The model under review builds one solid part; all positions refer to its coordinate system, in mm. Round coordinates to 2 decimals unless told otherwise and drop trailing zeros. Loops run counter-clockwise (first coordinate to the right, second up) from the corner with the lowest first, then second, coordinate; pieces in that order, holes last. Notation, with made-up numbers: M 62.25,35 L 94.25,35 A3 cw 94.25,40 Z; hole C -24.5,57.5 d5. An arc over 180 degrees is marked long. Answer as a JSON object with one key per item and string values. Group by question number.
Item 1: Consider section C-C (y = 2). Give the boundary of the cut face in (x, z).
Item 2: Consider section D-D (z = 5.4). Give the boundary of the cut face in (x, y) (3 decimals).
Item 3: Insertion check: P1, Ø1, axis at y = 5, z = 1, coming from the -X side; P2, Ø2, axis at y = 4.5, z = 1, coming from the +X side. Each pin has a flat end and moves straight along its axis. Give the tip position at first contact, or say it passes through.
Item 4: To check wall thickness, follow line 1 (Y direction, x = 20, z = 3.05); line 2 (X direction, y = -1.5, z = 0.9); line 3 (X direction, y = -1.25, z = 3.3). State the ranges of each line that lie inside material, in increasing order.
Item 5: Consider section B-B (z = 3.1). Give the boundary of the cut face in (x, y) (3 decimals).
Item 6: The part is to be moulded in two halves that separate along Y. For faces 1 (the face through (10.055, -1.684, 2.859)), 2 (the face through (-8.521, 0.035, 4.922)), 3 (the face through (27.229, 4.779, 5.114)), 4 (the face through (-8.5, -6.07, 2.01)), say which applies: +Y half, -Y half, draft (parallel to the pull), parting line (faces both ways), or undercut.
Item 7: Consider section A-A (y = 0). Give the boundary of the cut face in (x, z) (3 decimals).
Solid Edge part; units mm, degrees
sketch "Sketch1" plane through (0, 0, 0) normal (0, 0, 1) x (1, 0, 0)
  line L0 (-5, -7.5) -> (25, -7.5)
  arc A0 (25, -7.5) -> (30, -2.5) centre (25, -2.5) ccw
  line L1 (30, -2.5) -> (30, 2.5)
  arc A1 (25, 7.5) -> (30, 2.5) centre (25, 2.5) cw
  line L2 (25, 7.5) -> (-5, 7.5)
  arc A2 (-10, 2.5) -> (-5, 7.5) centre (-5, 2.5) cw
  line L3 (-10, 2.5) -> (-10, -2.5)
  arc A3 (-10, -2.5) -> (-5, -7.5) centre (-5, -2.5) ccw
  arc A4 (1.1832, 1.15) -> (-1.1832, 1.15) centre (0, 0) cw
  line L4 (0, 1.15) -> (-1.1832, 1.15)
  line L5 (0, 1.15) -> (1.1832, 1.15)
  arc A5 (11.2077, 1.175) -> (8.7923, 1.175) centre (10, 0) cw
  line L6 (10, 1.175) -> (8.7923, 1.175)
  line L7 (10, 1.175) -> (11.2077, 1.175)
  arc A6 (21.2042, 1.2) -> (18.7958, 1.2) centre (20, 0) cw
  line L8 (20, 1.2) -> (18.7958, 1.2)
  line L9 (20, 1.2) -> (21.2042, 1.2)
extrude "Protrusion1" add sketch "Sketch1" along normal blind 5.8
chamfer "Chamfer_top" distance 3 angle 30 8 edges at (28.5355, -6.0355, 5.8) (30, 0, 5.8) (28.5355, 6.0355, 5.8) (10, 7.5, 5.8) (-8.5355, 6.0355, 5.8) (-10, 0, 5.8) (-8.5355, -6.0355, 5.8) (10, -7.5, 5.8) measured on face at (-3.7333, -4.85, 5.8)
Geometry results:
{
 "1": {"outline": "M -10,0 L 30,0 L 30,4.07 L 27,5.8 L -7,5.8 L -10,4.07 Z"},
 "2": {"outline": "M -7.693,-2.5 A2.693 ccw -5,-5.193 L 25,-5.193 A2.693 ccw 27.693,-2.5 L 27.693,2.5 A2.693 ccw 25,5.193 L -5,5.193 A2.693 ccw -7.693,2.5 Z; hole M -1.183,1.15 A1.65 ccw long 1.183,1.15 L 0,1.15 Z; hole M 8.792,1.175 A1.685 ccw long 11.208,1.175 L 10,1.175 Z; hole M 18.796,1.2 A1.7 ccw long 21.204,1.2 L 20,1.2 Z"},
 "3": {"P1": "stops at x = -9.58", "P2": "stops at x = 29.9"},
 "4": {"line 1": "y = -7.5 to -1.7, 1.2 to 7.5", "line 2": "x = -10 to -0.69, 0.69 to 9.23, 10.77 to 19.2, 20.8 to 30", "line 3": "x = -10 to -1.08, 1.08 to 8.87, 11.13 to 18.85, 21.15 to 30"},
 "5": {"outline": "M -10,-2.5 A5 ccw -5,-7.5 L 25,-7.5 A5 ccw 30,-2.5 L 30,2.5 A5 ccw 25,7.5 L -5,7.5 A5 ccw -10,2.5 Z; hole M -1.183,1.15 A1.65 ccw long 1.183,1.15 L 0,1.15 Z; hole M 8.792,1.175 A1.685 ccw long 11.208,1.175 L 10,1.175 Z; hole M 18.796,1.2 A1.7 ccw long 21.204,1.2 L 20,1.2 Z"},
 "6": {"face 1": "undercut", "face 2": "draft", "face 3": "+Y half", "face 4": "-Y half"},
 "7": {"outline": "M -10,0 L -1.65,0 L -1.65,5.8 L -7,5.8 L -10,4.068 Z; M 1.65,0 L 8.315,0 L 8.315,5.8 L 1.65,5.8 Z; M 11.685,0 L 18.3,0 L 18.3,5.8 L 11.685,5.8 Z; M 21.7,0 L 30,0 L 30,4.068 L 27,5.8 L 21.7,5.8 Z"}
}
